Autodesk Inventor part; units mm, degrees
ref_plane "YZ Plane" through (0, 0, 0) normal (1, 0, 0) x (0, 1, 0)
ref_plane "XZ Plane" through (0, 0, 0) normal (0, 1, 0) x (-1, 0, 0)
ref_plane "XY Plane" through (0, 0, 0) normal (0, 0, 1) x (1, 0, 0)
sketch "Sketch1" plane through (0, 0, 0) normal (0, 0, 1) x (1, 0, 0)
  line L0 (254.7886, 18.124) -> (254.7886, 0) construction
  line L1 (192, 54.375) -> (254.7886, 18.124)
  line L2 (0, 0) -> (487.78, 0)
  line L3 (254.7886, 18.124) -> (256.7886, 18.124)
  line L4 (256.7886, 18.124) -> (327.1228, 36.97)
  line L5 (327.1228, 36.97) -> (327.1228, 0)
  line L6 (327.1228, 40.0758) -> (255.8936, 20.258)
  line L7 (255.8936, 20.258) -> (255.0924, 20.258)
  line L8 (255.0924, 20.258) -> (192.3194, 56.5)
  line L9 (327.1228, 36.97) -> (327.1228, 40.0758)
  line L10 (192, 54.375) -> (191.7835, 54.5)
  line L11 (0, 0) -> (0, 54.5)
  line L12 (0, 54.5) -> (274.8621, 54.5) construction
  line L13 (191.7835, 54.5) -> (188.7835, 54.5)
  line L14 (188.7835, 54.5) -> (188.7835, 56.5)
  line L15 (188.7835, 56.5) -> (192.3194, 56.5)
  line L16 (327.1228, 0) -> (327.1228, 59.5)
  line L17 (327.1228, 59.5) -> (323.1228, 59.5)
  line L18 (323.1228, 59.5) -> (323.1228, 38.9629)
  point P0 (322.4487, 38.7754)
  point P1 (191.9595, 55.4142)
  point P2 (188.9595, 55.4)
  dimension "d2" = 18.124
  dimension "d4" = 30
  dimension "d5" = 18.124
  dimension "d6" = 2
  dimension "d7" = 15
  dimension "d8" = 36.97
  dimension "d9" = 2
  dimension "d19" = 54.5
  dimension "d20" = 3
  dimension "d21" = 2
  dimension "d22" = 59.5
  dimension "d23" = 4
revolve "Revolution1" add sketch "Sketch1" angle 360 about axis through (0, 0, 0) along (1, 0, 0)
properties part number "stainless steel final nozzle" material "Stainless Steel"
Here's how the part is built. I have some questions about the finished solid (model axes, mm). A direction names the side the tool comes from. Round coordinates to 2 decimals unless told otherwise and drop trailing zeros. Loops run counter-clockwise (first coordinate to the right, second up) from the corner with the lowest first, then second, coordinate; pieces in that order, holes last. Notation, with made-up numbers: (47.25, 50) -> (72.25, 50) arc R30 ccw to (72.25, 83) -> close; hole circle Ø1 at (22, 4.5). An arc over 180 degrees is marked (long way). Answer as CSV lines item,"result".
1. For pin 1 (1 mm diameter, centred on x = 302.5, z = 0, fed in from +Y); pin 2 (2 mm diameter, centred on y = -41, z = 39, fed in from -X); pin 3 (3 mm diameter, centred on x = 214, z = 28, fed in from -Y); pin 4 (3 mm diameter, centred on y = 3.5, z = 47, fed in from -X), each with a flat end and sliding along its axis, tell me the tip position at first contact or that it passes through.
Final values:
pin 1,"stops at y = 33.36"
pin 2,"stops at x = 188.78"
pin 3,"stops at y = -35.54"
pin 4,"stops at x = 201.95"
2. If I drill on L1, parallel to Z at x = 255.45, y = 0; L2, parallel to Z at x = 190, y = 0; L3, parallel to X at y = -15.5, z = 48, over which ranges is the centre line in solid material (lowest first)?
Final values:
L1,"z = -20.26 to -18.12, 18.12 to 20.26"
L2,"z = -56.5 to -54.5, 54.5 to 56.5"
L3,"x = 198.81 to 202.81, 323.12 to 327.12"
3. If we section it at D-D on x = 246: Please give me the cut outline in (y, z) (1 decimal), plus the area to 3 significant figures.
Final values:
outline,"circle Ø51 at (0, 0); hole circle Ø46.4 at (0, 0)"
area,"353 mm^2"
4. Which directions (+Z, -Z, +X, -X, +Y, -Y) give clear straight access to the entire face, cutting with the end or side of a thin tool? Please do faces 1 (the face through (255.8, -14.38, -11.03)), 2 (the face through (237.216, -3.981, -30.319)), 3 (the face through (190.576, 30.374, 47.641)).
Final values:
face 1,"+X, -X"
face 2,"none"
face 3,"-X"
5. Thinking about a two-plate mould opening in X: for faces 4 (the face through (188.784, -30, 46)), 5 (the face through (323.123, 12, -39)), 6 (the face through (325.09, 31.99, -50.17)), which applies, released by +X, released by -X, zero draft, split by the parting line, or undercut?
Final values:
face 4,"released by -X"
face 5,"undercut"
face 6,"zero draft"
6. If we section it at C-C on x = 270.5: Please give me the cut outline in (y, z).
Final values:
outline,"circle Ø48.64 at (0, 0); hole circle Ø43.6 at (0, 0)"
